from build123d import *

# Parameters (mm, degrees)
SZKIC2_R                    = 22.5
DODANIE_WYCI_GNI_CIE1_DEPTH = 1
SZKIC3_R                    = 21.5
DODANIE_WYCI_GNI_CIE2_DEPTH = 7.5
WYTNIJ_WYCI_GNI_CIE1_DEPTH  = 10


with BuildPart() as part:
    # Szkic2 → Dodanie-wyciągnięcie1 (new body)
    with BuildSketch(Plane.XY):
        Circle(SZKIC2_R)
    extrude(amount=DODANIE_WYCI_GNI_CIE1_DEPTH)

    # Szkic3 → Dodanie-wyciągnięcie2 (add)
    with BuildSketch(Plane.XY.offset(1)):
        Circle(SZKIC3_R)
    extrude(amount=DODANIE_WYCI_GNI_CIE2_DEPTH)

    # Szkic4 → Wytnij-wyciągnięcie1 (cut)
    with BuildSketch(Plane.XY.offset(8.5)):
        with BuildLine():
            Line((-1, -9.949874371), (-1, -23.658625842))
            Line((-1, -23.658625842), (1, -23.658625842))
            Line((1, -23.658625842), (1, -9.949874371))
            ThreePointArc((1, -9.949874371), (0, 10), (-1, -9.949874371))
        make_face()
    extrude(amount=-WYTNIJ_WYCI_GNI_CIE1_DEPTH, mode=Mode.SUBTRACT)


solid = part.part
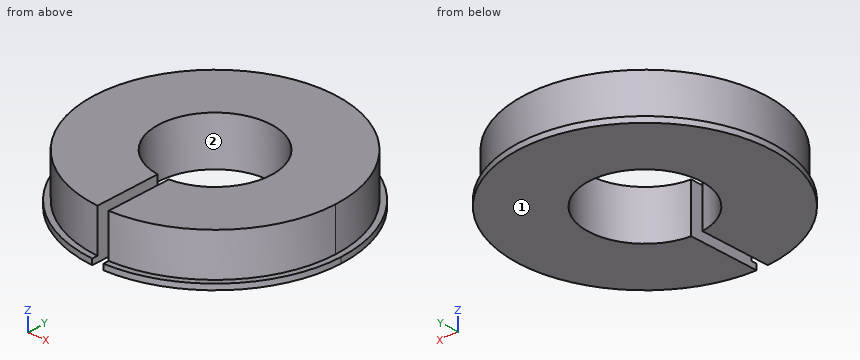
The model under review builds one solid part; all positions refer to its coordinate system, in mm. Face numbers are marked on the shaded views. Coordinates: 2 decimals unless noted, no trailing zeros. Loops run counter-clockwise (first coordinate to the right, second up) from the corner with the lowest first, then second, coordinate; pieces in that order, holes last. Notation, with made-up numbers: M 10,1.25 L 15,1.25 A7 ccw 15,6.25 Z; hole C 18,44.25 d11. An arc over 180 degrees is marked long. Put each result on its own line as item: value. Start each with the question number.
Q1. Clearance check with flat-ended pins moving along their axes: pin 1 (4 mm diameter, centred on y = -14.5, z = 3, fed in from +X); pin 2 (1.5 mm diameter, centred on x = -12.5, z = 7, fed in from +Y); pin 3 (6 mm diameter, centred on x = -6.5, y = -10, fed in from -Z); pin 4 (5 mm diameter, centred on y = 12, z = 7, fed in from +X). State where each tip first meets the part, or that it passes through.
Q2. Wall thickness on line 1 (X direction, y = 0, z = 5.25); line 2 (Y direction, x = 6, z = 4.75); line 3 (Y direction, x = -4.5, z = 0.75): over which ranges is each line inside the solid? List them lowest first.
Q3. Add section D-D (x = 17.5). Write out the cut boundary in (y, z), and give its area (3 significant figures).
Q4. Add section C-C (z = 5.5). Write out the cut boundary in (x, y), and give its area (3 significant figures).
Q5. The part is to be moulded in two halves that separate along X. For the marked faces 1 and 2, say which applies: +X half, -X half, draft (parallel to the pull), parting line (faces both ways), or undercut.
Q6. Add section B-B (y = -2.5). Write out the cut boundary in (x, z).
Q7. Add section A-A (x = -2). Write out the cut boundary in (y, z).
Answers:
1. pin 1: stops at x = 17.49
1. pin 2: stops at y = 18.01
1. pin 3: stops at z = 0
1. pin 4: stops at x = 19.29
2. line 1: x = -21.5 to -10, 10 to 21.5
2. line 2: y = -20.65 to -8, 8 to 20.65
2. line 3: y = -22.05 to -8.93, 8.93 to 22.05
3. outline: M -14.14,0 L 14.14,0 L 14.14,1 L 12.49,1 L 12.49,8.5 L -12.49,8.5 L -12.49,1 L -14.14,1 Z
3. area: 216 mm^2
4. outline: M -1,-21.48 L -1,-9.95 A10 cw long 1,-9.95 L 1,-21.48 A21.5 ccw long Z
4. area: 1,120 mm^2
5. face 1: draft
5. face 2: undercut
6. outline: M -22.36,0 L -9.68,0 L -9.68,8.5 L -21.35,8.5 L -21.35,1 L -22.36,1 Z; M 9.68,0 L 22.36,0 L 22.36,1 L 21.35,1 L 21.35,8.5 L 9.68,8.5 Z
7. outline: M -22.41,0 L -9.8,0 L -9.8,8.5 L -21.41,8.5 L -21.41,1 L -22.41,1 Z; M 9.8,0 L 22.41,0 L 22.41,1 L 21.41,1 L 21.41,8.5 L 9.8,8.5 Z
